Autodesk Inventor part; units mm, degrees
ref_plane "Work Plane1" through (6.4515, 0, 0) normal (0, 0.866, -0.5) x (-1, 0, 0)
ref_plane "YZ Plane" through (0, 0, 0) normal (1, 0, 0) x (0, 1, 0)
ref_plane "XZ Plane" through (0, 0, 0) normal (0, 1, 0) x (-1, 0, 0)
sketch "Sketch1" plane through (0, 0, 0) normal (1, 0, 0) x (0, 1, 0)
  line L0 (-4.6188, -8) -> (-9.2376, 0)
  line L1 (-9.2376, 0) -> (-4.6188, 8)
  line L2 (-4.6188, 8) -> (4.6188, 8)
  line L3 (4.6188, 8) -> (9.2376, 0)
  line L4 (9.2376, 0) -> (4.6188, -8)
  line L5 (4.6188, -8) -> (-4.6188, -8)
  point P0 (0, 0)
  point P1 (0, 0)
  dimension "d0" = 18.4752
extrude "Body" add sketch "Sketch1" along normal blind 8
sketch "Sketch2" plane through (0, 0, 0) normal (0, 0, 1) x (1, 0, 0)
  line L0 (8, 0) -> (18, 0)
  arc A0 (18, 0) -> (10.5, 7.5) centre (10.5, 0) ccw
  line L1 (10.5, 7.5) -> (8, 7.5)
  line L2 (8, -4.6188) -> (8, 4.6188)
  line L3 (8, 0) -> (8, 7.5)
  line L4 (5.6893, 0) -> (21.864, 0)
  dimension "d8" = 7.5
  dimension "d9" = 10
revolve "Cap" add sketch "Sketch2" angle 360 about axis through (8, 0, 0) along (1, 0, 0)
sketch "Sketch3" plane through (0, 0, 0) normal (-1, 0, 0) x (0, 0, 1)
  line L0 (0, -12.9326) -> (0, 12.9326)
  line L1 (-11.2, 0) -> (11.2, 0)
  point P0 (0, 0)
hole "Thread" at (0, 0, 0) direction (1, 0, 0) diameter 8.376 depth 12.903 tip angle 120
sketch "Sketch4" plane through (0, 0, 0) normal (0, 0, 1) x (1, 0, 0)
  line L0 (0, 4.6188) -> (0, 9.2376)
  line L1 (0, 9.2376) -> (8, 9.2376)
  line L2 (8, 4.6188) -> (8, 9.2376)
  line L3 (-1.6, 0) -> (9.6, 0)
  line L4 (1.1187, 9.2376) -> (0, 7.3)
  line L5 (7.2855, 9.2376) -> (8, 8)
  dimension "d3" = 14.6
  dimension "d4" = 30
  dimension "d5" = 16
  dimension "d6" = 30
revolve "Chamfer1" cut sketch "Sketch4" angle 360 about axis through (-10, 0, 0) along (1, 0, 0)
chamfer "Chamfer2" distance 0.8119 angle 30 1 edges at (0, 0, -4.188) measured on face at (0, 6.1818, -0.7506)
ref_plane "Work Plane1" through (6.4515, 0, 0) normal (0, 0.866, -0.5) x (-1, 0, 0)
equation "\"d0\" = 1.1547 * SW"
equation "\"d1\" = SIH"
equation "\"d8\" = KR"
equation "\"d9\" = KOH1 - SIH"
equation "\"d11\" = GEL"
equation "\"d12\" = 1.02 * GEL"
equation "\"d3\" = SW0"
equation "\"d4\" = ANG1"
equation "\"d5\" = SW01"
equation "\"d6\" = ANG2"
equation "\"d14\" = -0.5 * GD1 + 0.5 * NND"
equation "\"d36\" = -0.5 * GD1 + 0.5 * NND"
equation "\"ANG1\" = 30deg"
equation "\"ANG2\" = 30deg"
equation "\"SIH\" = 8"
equation "\"KOH1\" = 18"
equation "\"GEL\" = 12.65"
equation "\"SW\" = 16"
equation "\"KR\" = 7.5"
equation "\"SW0\" = 14.6"
equation "\"SW01\" = SW"
equation "\"GUL\" = 0.541266 * PTC"
equation "\"TOA\" = 30deg"
equation "\"PTC\" = 1.5"
equation "\"E0\" = 1.155 * SW"
equation "\"GAL\" = 0.541266 * PTC"
properties part number "M10 DN A2" material "Stainless Steel AISI 304"
Could you check a few things on this model? Use its own coordinates, in mm. A direction names the side the tool comes from. Give positions to 0.01 mm unless a question says otherwise; leave off trailing zeros. Write each loop counter-clockwise with the first axis right and the second up, starting at its lowest first coordinate (ties: lowest second). Pieces come first, ordered by that corner, then holes. Notation, with made-up numbers: (15, 34.5) - (23, 34.5) arc R19 ccw to (23, 47.5) - close; hole circle Ø3 at (35, -12). An arc over 180 degrees is marked (long way). One line per item, written item: value. Start each with the question number.
Item 1: If we mould it in two halves opening along Z, with no side actions, what happens to faces 1 (the face through (14.9, -0.7, -0.2)), 2 (the face through (9.232, -7.493, -0.33)), 3 (the face through (4.149, -6.896, -4.056)), 4 (the face through (4.149, -6.961, 3.944))? For each: +Z half, -Z half, draft (parallel to the pull), parting line (faces both ways), or undercut.
Item 2: Imagine slicing it at C-C, the plane x = 15. List the corners of the cut face in (y, z) for me.
Item 3: I'm going to push flat-ended pins straight in: pin 1 (2 mm diameter, centred on y = -7.5, z = -2, fed in from +X); pin 2 (1.5 mm diameter, centred on x = 7.5, y = -5.5, fed in from +Z); pin 3 (3 mm diameter, centred on x = 5, z = 6.5, fed in from -Y). Where does each tip first touch, or does it pass through?
Item 4: Please list where these lines run through material, in increasing order: line 1 (Z direction, x = 4.5, y = 0); line 2 (Z direction, x = 9.75, y = 0); line 3 (Y direction, x = 10.75, z = 1.75). Write a range as from..to.
Item 5: Imagine slicing it at B-B, the plane x = 9.25. List the corners of the cut face in (y, z) for me.
Item 6: Which directions (+Z, -Z, +X, -X, +Y, -Y) give clear straight access to the entire face, cutting with the end or side of a thin tool? Please do faces 5 (the face through (8, 5, -6)), 6 (the face through (6.773, -2.83, -3.087)), 7 (the face through (4.149, 6.896, 4.056)).
Item 7: Imagine slicing it at A-A, the plane x = 5.75. List the corners of the cut face in (y, z) for me, and give its area (3 significant figures).
Geometry says:
1. face 1: undercut
1. face 2: parting line
1. face 3: -Z half
1. face 4: +Z half
2. outline: circle Ø12 at (0, 0); hole circle Ø1.11 at (0, 0)
3. pin 1: x = 13.74
3. pin 2: z = 7.75
3. pin 3: y = -6.35
4. line 1: -8..-4.19, 4.19..8
4. line 2: -7.5..-4.19, 4.19..7.5
4. line 3: -7.29..-3.8, 3.8..7.29
5. outline: circle Ø15 at (0, 0); hole circle Ø8.38 at (0, 0)
6. face 5: +X
6. face 6: -X
6. face 7: +Z, +X, -X, +Y
7. outline: (-9.24, 0) - (-4.62, -8) - (4.62, -8) - (9.24, 0) - (4.62, 8) - (-4.62, 8) - close; hole circle Ø8.38 at (0, 0)
7. area: 167 mm^2
